CAD build for the part. Positions are in the model's coordinates, mm. A direction names the side the tool comes from. Round coordinates to 2 decimals unless told otherwise and drop trailing zeros. Write each loop counter-clockwise with the first axis right and the second up, starting at its lowest first coordinate (ties: lowest second). Pieces come first, ordered by that corner, then holes. Notation, with made-up numbers: (30, -26) -> (88, -26) arc R6 ccw to (88, -17) -> close; hole circle Ø8 at (76.25, 55). An arc over 180 degrees is marked (long way). Put each result on its own line as item: value. Start each with the question number.
1. Saw through at B-B on y = 1.6. State how many separate pieces and enclosed holes the cut face has, and give its area (3 significant figures).
2. Drill centre lines: line 1 (Z direction, x = 7, y = 2.35); line 2 (X direction, y = 2.15, z = 0); line 3 (X direction, y = 1.2, z = 18.5). Where is each one in solid material? Low to high. Write a range as from..to.
3. Saw through at A-A on z = 0. List the corners of the cut face in (x, y).
4. Flat gauge pins, fed straight in: P1, Ø0.9, axis at x = -5.5, y = 2, coming from the -Z side; P2, Ø1, axis at x = 27, y = 0.5, coming from the +Z side. Where does each tip first touch, or does it go through?
5. 3-axis set-ups, long thin cutter, end or side, ignore diameter. For faces 1 (the flat face through (-18, 2, -13)), 2 (the flat face through (25, 1, -23.5)), 3 (the cylindrical face through (34.797, 1.479, -16.641)), 4 (the cylindrical face through (-4.25, 1.52, -0.07)), 5 (the flat face through (-34, 1, 0)): which of +Z, -Z, +X, -X, +Y, -Y reach the whole face in a straight line?
6. Saw through at C-C on z = -25.5. List the corners of the cut face in (x, y).
from build123d import *

# Parameters (mm, degrees)
CROQUIS1_W              = 72
CROQUIS1_H              = 47
SALIENTE_EXTRUIR1_DEPTH = 3
CROQUIS3_W              = 13
CROQUIS3_H              = 10
CROQUIS3_W_2            = 2
CROQUIS3_H_2            = 21
CORTAR_EXTRUIR2_DEPTH   = 44.095823464
CROQUIS2_R              = 1.6
CORTAR_EXTRUIR1_DEPTH   = 44.095823464
CORTAR_EXTRUIR3_DEPTH   = 34.75
CROQUIS5_R              = 1.6
CORTAR_EXTRUIR7_DEPTH   = 10
CHAFL_N1_SIZE           = 2.5
REDONDEO2_R             = 1
CROQUIS6_R              = 1.6
SALIENTE_EXTRUIR2_DEPTH = 3
REDONDEO1_R             = 4


# Some blends are built 0.0001 mm under size
with BuildPart() as part:
    # Croquis1 → Saliente-Extruir1 (new body)
    with BuildSketch(Plane(origin=(0, 0, 0), x_dir=(1, 0, 0), z_dir=(0, 1, 0))):
        Rectangle(CROQUIS1_W, CROQUIS1_H)
    extrude(amount=SALIENTE_EXTRUIR1_DEPTH)

    # Croquis3 → Cortar-Extruir2 (cut, through all)
    with BuildSketch(Plane(origin=(0, 3, 0), x_dir=(1, 0, 0), z_dir=(0, 1, 0))):
        Polygon((-8, 13), (-8, 10), (-3, 10), (-3, 15.5), (15, 15.5), (15, 23.5), (-36, 23.5), (-36, 19.5), (-28, 19.5), (-28, 13), align=None)
        Polygon((-28, -13), (-8, -13), (-8, -10), (-3, -10), (-3, -15.5), (28, -15.5), (28, -23.5), (-36, -23.5), (-36, -19.5), (-28, -19.5), align=None)
        with Locations((29.5, 10.5)):
            Rectangle(CROQUIS3_W, CROQUIS3_H)
        with Locations((-35, 0)):
            Rectangle(CROQUIS3_W_2, CROQUIS3_H_2)
    extrude(amount=-CORTAR_EXTRUIR2_DEPTH, mode=Mode.SUBTRACT)

    # Croquis2 → Cortar-Extruir1 (cut, through all)
    with BuildSketch(Plane(origin=(0, 3, 0), x_dir=(1, 0, 0), z_dir=(0, 1, 0))):
        with Locations((-32, 19.5)):
            Circle(CROQUIS2_R)
        with Locations(Location((32, 19.5, 0), (0, 0, 270))):
            Circle(CROQUIS2_R)
        with Locations(Location((32, -19.5, 0), (0, 0, 270))):
            Circle(CROQUIS2_R)
        with Locations((-32, -19.5)):
            Circle(CROQUIS2_R)
    extrude(amount=-CORTAR_EXTRUIR1_DEPTH, mode=Mode.SUBTRACT)

    # Croquis4 → Cortar-Extruir3 (cut)
    with BuildSketch(Plane(origin=(0, 3, 0), x_dir=(1, 0, 0), z_dir=(0, 1, 0))):
        with BuildLine():
            Line((-1.25, -3), (11.75, -3))
            Line((11.75, -3), (11.75, 3))
            Line((11.75, 3), (-1.25, 3))
            ThreePointArc((-1.25, 3), (-4.25, 0), (-1.25, -3))
        make_face()
    extrude(amount=-CORTAR_EXTRUIR3_DEPTH, mode=Mode.SUBTRACT)

    # Croquis5 → Cortar-Extruir7 (cut)
    with BuildSketch(Plane(origin=(0, 3, -3), x_dir=(1, 0, 0), z_dir=(0, -1, 0))):
        with Locations(Location((-30, 13, 0), (0, 0, 270))):
            Circle(CROQUIS5_R)
        with Locations(Location((-30, -7, 0), (0, 0, 270))):
            Circle(CROQUIS5_R)
        with Locations(Location((-10, 13, 0), (0, 0, 270))):
            Circle(CROQUIS5_R)
        with Locations(Location((-10, -7, 0), (0, 0, 270))):
            Circle(CROQUIS5_R)
    extrude(amount=CORTAR_EXTRUIR7_DEPTH, mode=Mode.SUBTRACT)

    # Chaflán1
    # the kernel refuses this chamfer: 2.5 mm, written as the material it takes off along each edge
    with BuildSketch(Plane(origin=(-36, 9.42920747, 10.5), x_dir=(-0.0274958766105877, 0, 0.9996219169112968), z_dir=(0, -1, 0))) as chafl_n1_piece_1_section:
        Polygon((CHAFL_N1_SIZE * 0.999621916911, -CHAFL_N1_SIZE * 0.0274958766106), (-CHAFL_N1_SIZE * 0.0274958766106, -CHAFL_N1_SIZE * 0.999621916911), (0, 0), align=None)
    chafl_n1_piece_1 = extrude(amount=15.85841494, mode=Mode.PRIVATE)
    chafl_n1_piece_1 = split(chafl_n1_piece_1, bisect_by=Plane(origin=(-34, 1.5, 11.364296031), z_dir=(-1, 0, 0)), keep=Keep.TOP, mode=Mode.PRIVATE)
    add(chafl_n1_piece_1, mode=Mode.SUBTRACT)
    with BuildSketch(Plane(origin=(-36, 9.42920747, -10.5), x_dir=(0.9996219169112968, 0, 0.027495876610586282), z_dir=(0, -1, 0))) as chafl_n1_piece_2_section:
        Polygon((CHAFL_N1_SIZE * 0.999621916911, -CHAFL_N1_SIZE * 0.0274958766106), (-CHAFL_N1_SIZE * 0.0274958766106, -CHAFL_N1_SIZE * 0.999621916911), (0, 0), align=None)
    chafl_n1_piece_2 = extrude(amount=15.85841494, mode=Mode.PRIVATE)
    chafl_n1_piece_2 = split(chafl_n1_piece_2, bisect_by=Plane(origin=(-34, 1.5, -11.364296031), z_dir=(-1, 0, 0)), keep=Keep.TOP, mode=Mode.PRIVATE)
    add(chafl_n1_piece_2, mode=Mode.SUBTRACT)

    # Redondeo2
    redondeo2_edges = [part.edges().sort_by_distance(p)[0] for p in [
        (11.75, 1.5, -3),
        (11.75, 1.5, 3),
        (-36, 1.5, 13),
        (-36, 1.5, -13),
        (-34, 1.5, 11),
        (-34, 1.5, -11),
        (-8, 1.5, -13),
        (-28, 1.5, -13),
        (-3, 1.5, -15.5),
        (-3, 1.5, -10),
        (-8, 1.5, -10),
        (-28, 1.5, 13),
        (-8, 1.5, 13),
        (-8, 1.5, 10),
        (-3, 1.5, 10),
        (-3, 1.5, 15.5),
        (23, 1.5, -5.5),
        (23, 1.5, -15.5),
    ]]
    fillet(redondeo2_edges, radius=REDONDEO2_R)

    # Croquis6 → Saliente-Extruir2 (add, through all)
    with BuildSketch(Plane(origin=(0, 3, 0), x_dir=(1, 0, 0), z_dir=(0, 1, 0))):
        with BuildLine():
            ThreePointArc((-34.197424136, -29.570815068), (-29.673479987, -25.412473854), (-28, -19.500000848))
            ThreePointArc((-28, -19.500000848), (-31.999999152, -15.5), (-36, -19.499999152))
            ThreePointArc((-36, -19.499999152), (-36.48674652, -21.219694449), (-37.802575864, -22.429184932))
            ThreePointArc((-37.802575864, -22.429184932), (-39.570815068, -27.802575864), (-34.197424136, -29.570815068))
        make_face()
        with Locations(Location((-36, -26, 0), (0, 0, 270))):
            Circle(CROQUIS6_R, mode=Mode.SUBTRACT)
        with Locations(Location((-32, -19.5, 0), (0, 0, 270))):
            Circle(CROQUIS6_R, mode=Mode.SUBTRACT)
    saliente_extruir2 = extrude(amount=-SALIENTE_EXTRUIR2_DEPTH)

    # Simetría1: Saliente-Extruir2 across plane
    add(saliente_extruir2.mirror(Plane.XY))

    # Redondeo1
    redondeo1_edges = [part.edges().sort_by_distance(p)[0] for p in [
        (36, 1.5, -23.5),
        (36, 1.5, 23.5),
        (15, 1.5, -23.5),
        (15, 1.5, -15.5),
        (28, 1.5, 15.5),
        (36, 1.5, -5.5),
        (36, 1.5, -15.5),
        (28, 1.5, 23.5),
    ]]
    fillet(redondeo1_edges, radius=REDONDEO1_R - 0.0001)  # a hair under: the kernel refuses the full size


solid = part.part
Return value:
1. separate pieces: 1
1. enclosed holes: 11
1. area: 2,190 mm^2
2. line 1: z = -15.5..-3, 3..15.5
2. line 2: x = -34..-4.25, 11.75..36
2. line 3: x = -36..-33.25, -30.75..-28, 27.87..30.75, 33.25..36
3. outline: (-34, 0) -> (-4.25, 0) -> (-4.25, 3) -> (-34, 3) -> close; (11.75, 0) -> (36, 0) -> (36, 3) -> (11.75, 3) -> close
4. P1: stops at z = -10
4. P2: stops at z = 17.56
5. face 1: -Z, +Y, -Y
5. face 2: -Z, +X, +Y, -Y
5. face 3: +X, +Y, -Y
5. face 4: +Y, -Y
5. face 5: -X, +Y, -Y
6. outline: (-39.97, 0) -> (-37.52, 0) -> (-37.52, 3) -> (-39.97, 3) -> close; (-34.48, 0) -> (-29.73, 0) -> (-29.73, 3) -> (-34.48, 3) -> close
